Geometry: final body of the model. Coordinates: model frame, mm. A direction names the side the tool comes from. Give positions to 0.01 mm unless a question says otherwise; leave off trailing zeros. Loops run counter-clockwise (first coordinate to the right, second up) from the corner with the lowest first, then second, coordinate; pieces in that order, holes last.
from build123d import *

# Parameters (mm, degrees)
BOSS_EXTRUDE1_DEPTH = 30
CUT_EXTRUDE1_START  = -3
CUT_EXTRUDE1_DEPTH  = 79


with BuildPart() as part:
    # Sketch1 → Boss-Extrude1 (new body)
    with BuildSketch(Plane.XY):
        with BuildLine():
            Line((3, 47), (82, 47))
            ThreePointArc((82, 47), (84.121320344, 46.121320344), (85, 44))
            Line((85, 44), (85, -3))
            ThreePointArc((85, -3), (84.121320344, -0.878679656), (82, 0))
            Line((82, 0), (3, 0))
            ThreePointArc((3, 0), (0.878679656, -0.878679656), (0, -3))
            Line((0, -3), (0, 44))
            ThreePointArc((0, 44), (0.878679656, 46.121320344), (3, 47))
        make_face()
    extrude(amount=BOSS_EXTRUDE1_DEPTH)

    # Sketch2 → Cut-Extrude1 (cut)
    with BuildSketch(Plane(origin=(85, 0, 0), x_dir=(0, 0, -1), z_dir=(1, 0, 0)).offset(CUT_EXTRUDE1_START)):
        with BuildLine():
            Line((-30, 3), (-11.5, 3))
            ThreePointArc((-11.5, 3), (-3.066269455, 10.440665731), (-9.397849462, 19.735955507))
            ThreePointArc((-9.397849462, 19.735955507), (-9.831775106, 20.020329144), (-10, 20.511104261))
            Line((-10, 20.511104261), (-10, 20.58947854))
            ThreePointArc((-10, 20.58947854), (-9.881909085, 21.007808553), (-9.5625, 21.302636131))
            ThreePointArc((-9.5625, 21.302636131), (-3.330202092, 34.795678233), (-15, 44))
            Line((-15, 44), (-30, 44))
            Line((-30, 44), (-30, 3))
        make_face()
    extrude(amount=-CUT_EXTRUDE1_DEPTH, mode=Mode.SUBTRACT)


solid = part.part
Item 1: Section query A-A on z = 19.5. Return loops of the section in (x, y), plus the area to 3 significant figures.
Values follow:
outline: (0, -3) arc R3 cw to (3, 0) - (82, 0) arc R3 cw to (85, -3) - (85, 44) arc R3 ccw to (82, 47) - (3, 47) arc R3 ccw to (0, 44) - close; hole (3, 3) - (82, 3) - (82, 44) - (3, 44) - close
area: 756 mm2
Item 2: Section query B-B on x = 26. Return loops of the section in (y, z), plus the area to 3 significant figures.
Values follow:
outline: (0, 0) - (47, 0) - (47, 30) - (44, 30) - (44, 15) arc R12 cw to (21.3, 9.56) arc R0.8 ccw to (20.59, 10) - (20.51, 10) arc R0.8 ccw to (19.74, 9.4) arc R8.5 cw to (3, 11.5) - (3, 30) - (0, 30) - close
area: 394 mm2
Item 3: Section query D-D on y = 34. Return loops of the section in (x, z).
Values follow:
outline: (0, 0) - (85, 0) - (85, 30) - (82, 30) - (82, 3.17) - (3, 3.17) - (3, 30) - (0, 30) - close
Item 4: Draft query along X for faces 1 (the face through (3, 24, 17)), 2 (the face through (43, 22, 0)), 3 (the face through (84.1, 46.14, 14.79)). Return one class per face: +X half, -X half, draft (parallel to the pull), parting line (faces both ways), or undercut.
Values follow:
face 1: undercut
face 2: draft
face 3: +X half
Item 5: Pin query (flat end, axial travel): pin 1 (9 mm diameter, centred on x = 45.5, z = 21.5, fed in from -Y); pin 2 (12 mm diameter, centred on x = 25.5, y = 27.5, fed in from +Z); pin 3 (2 mm diameter, centred on x = 73, y = 3.5, fed in from -Z). Return the tip coordinate at first contact, or that it passes through.
Values follow:
pin 1: stops at y = 0
pin 2: stops at z = 9.19
pin 3: stops at z = 0
Item 6: Set-up query: faces 4 (the face through (43, 44, 22)), 5 (the face through (84.14, -0.9, 14.79)), 6 (the face through (0.86, 46.1, 14.79)). Return all of +Z, -Z, +X, -X, +Y, -Y with unobstructed straight access to the full face (end or side cutting, diameter ignored); none if empty.
Values follow:
face 4: +Z
face 5: +Z, -Z, -Y
face 6: +Z, -Z, -X, +Y
Item 7: Ray query, probe 1 along X at (y, z) = (12, 27.75); probe 2 along Y at (x, z) = (18.5, 27.75); probe 3 along Y at (x, z) = (64, 4). Return the intervals inside material, ascending.
Values follow:
probe 1: x = 0 to 3, 82 to 85
probe 2: y = 0 to 3, 44 to 47
probe 3: y = 0 to 7.5, 15.5 to 27.2, 36.8 to 47
Item 8: Section query C-C on z = 4.75. Return loops of the section in (x, y).
Values follow:
outline: (0, -3) arc R3 cw to (3, 0) - (82, 0) arc R3 cw to (85, -3) - (85, 44) arc R3 ccw to (82, 47) - (3, 47) arc R3 ccw to (0, 44) - close; hole (3, 6.33) - (82, 6.33) - (82, 16.67) - (3, 16.67) - close; hole (3, 25.76) - (82, 25.76) - (82, 38.24) - (3, 38.24) - close
